Autodesk Inventor part; units mm, degrees
ref_plane "YZ Plane" through (0, 0, 0) normal (1, 0, 0) x (0, 1, 0)
ref_plane "XZ Plane" through (0, 0, 0) normal (0, 1, 0) x (-1, 0, 0)
ref_plane "XY Plane" through (0, 0, 0) normal (0, 0, 1) x (1, 0, 0)
sketch "Sketch1" plane through (0, 0, 0) normal (0, 0, 1) x (1, 0, 0)
  circle A0 centre (0, 0) radius 3.175
  circle A1 centre (0, 0) radius 1.5875
  line L0 (0, -3.175) -> (-19.05, -3.175)
  line L1 (-19.05, -3.175) -> (-19.05, 0)
  line L2 (-19.05, 0) -> (-1.5875, 0)
  line L3 (0, -1.5875) -> (0, -3.175)
  dimension "d0" = 6.35
  dimension "d1" = 3.175
  dimension "d2" = 19.05
  dimension "d3" = 3.175
extrude "Extrusion1" add sketch "Sketch1" along normal blind 25.4 contours L3 A1 L2 A0 | L0 L1 L2 A0 | A0 L2 A1 L3
sketch "Sketch2" plane through (-19.05, -3.175, 0) normal (0, -1, 0) x (1, 0, 0)
  line L0 (15.875, 15.875) -> (22.225, 15.875)
  line L1 (22.225, 15.875) -> (22.225, 9.525)
  line L2 (22.225, 9.525) -> (15.875, 9.525)
  line L3 (15.875, 9.525) -> (15.875, 15.875)
  line L4 (15.875, 25.4) -> (22.225, 25.4)
  circle A0 centre (6.35, 19.05) radius 1.5875
  circle A1 centre (6.35, 6.35) radius 1.5875
  point P0 (19.05, 0)
  point P1 (0, 25.4)
  point P2 (0, 0)
  dimension "d6" = 6.35
  dimension "d7" = 3.175
  dimension "d8" = 6.35
  dimension "d9" = 9.525
  dimension "d12" = 12.7
  dimension "d13" = 6.35
  dimension "d14" = 3.175
  dimension "d15" = 3.175
  dimension "d16" = 6.35
extrude "Extrusion2" cut sketch "Sketch2" against normal blind 25.4
properties part number "hinge two prong"
Verification items for the finished model (mm, model axes). A direction names the side the tool comes from. Round coordinates to 2 decimals unless told otherwise and drop trailing zeros. Order: outer loops, then holes, each group sorted by start corner. A loop starts at its lowest first (then second) coordinate and runs counter-clockwise, first axis right, second up. Notation, with made-up numbers: (-21, 65) -> (29, 65) arc R28 ccw to (29, 88) -> close; hole circle Ø3 at (53, 88). An arc over 180 degrees is marked (long way). Put each result on its own line as item: value.
1) Depth check by flat-ended pin: pin 1 (1.5 mm diameter, centred on y = 1.5, z = 7.5, fed in from -X); pin 2 (2 mm diameter, centred on y = -2, z = 4, fed in from +X); pin 3 (1.5 mm diameter, centred on y = -1, z = 22, fed in from +X). Enter the tip coordinate at first touch or a pass-through.
Final values:
pin 1: stops at x = -3.09
pin 2: stops at x = 3.01
pin 3: stops at x = 3.17
2) Section check A-A (z = 6.35). Give the number of separate pieces and of enclosed holes in the cut face, then the cut area to 3 significant figures.
Final values:
separate pieces: 2
enclosed holes: 1
area: 66.2 mm^2
3) Material ranges on line 1 (Y direction, x = 0, z = 21) (1 decimal); line 2 (Z direction, x = -13.5, y = -2.25); line 3 (Y direction, x = -10.5, z = 20) (3 decimals), recorded low to high.
Final values:
line 1: y = -3.2 to -1.6, 1.6 to 3.2
line 2: z = 0 to 4.98, 7.72 to 17.68, 20.42 to 25.4
line 3: y = -3.175 to 0
4) Mould release check, pull along Y, two halves, no side actions. Record for faces 1 (the flat face through (-1.4, -1.5, 9.525)), 2 (the cylindrical face through (-0.34, 1.55, 20.57)), 3 (the cylindrical face through (2.17, 2.32, 4.7)), 4 (the cylindrical face through (-0.34, 1.55, 4.7)): +Y half, -Y half, draft (parallel to the pull), parting line (faces both ways), or undercut.
Final values:
face 1: draft
face 2: undercut
face 3: parting line
face 4: undercut
5) Section check D-D (z = 14). Record the cut outline in (x, y) (3 decimals), then the cut area to 3 significant figures.
Final values:
outline: (-19.05, -3.175) -> (-3.175, -3.175) -> (-3.175, 0) -> (-19.05, 0) -> close
area: 50.4 mm^2
6) Set-up check for faces 5 (the flat face through (-11, 0, 13)), 6 (the cylindrical face through (2.17, 2.32, 20.57)), 7 (the flat face through (-3.175, -2, 13)): record each of +Z, -Z, +X, -X, +Y, -Y from which the full face is reachable in a straight line by a thin tool's end or side.
Final values:
face 5: +Z, -Z, -X, +Y
face 6: +Z, -Z
face 7: +X, +Y, -Y
